Could you check a few things on this model? Use its own coordinates, in mm. A direction names the side the tool comes from. Give positions to 0.01 mm unless a question says otherwise; leave off trailing zeros. Loops run counter-clockwise (first coordinate to the right, second up) from the corner with the lowest first, then second, coordinate; pieces in that order, holes last. Notation, with made-up numbers: (-2.75, 61.5) - (12.25, 61.5) arc R19 ccw to (12.25, 98.5) - close; hole circle Ø6 at (50.25, -17.5). An arc over 180 degrees is marked (long way). Write each question's results on one line, items separated by ' | '. Start each with the question number.
(1) Suppose I cut it at B-B (z = 57.5). Please give me the cut outline in (x, y).
(2) Suppose I cut it at C-C (y = -56). Please give me the cut outline in (x, z).
(3) On a 3-axis mill with a long thin cutter (end or side, diameter ignored), from which of +Z, -Z, +X, -X, +Y, -Y can I reach the whole of each face in a straight line? I mean faces 4 (the face through (139.692, -45.148, 38.633)), 5 (the face through (-2, -88.9, 38)). Say none if no direction works.
(4) Suppose I cut it at A-A (x = -48.5). Please give me the cut outline in (y, z), and give its area (3 significant figures).
(5) For pin 1 (5 mm diameter, centred on y = -68.5, z = 16, fed in from -X); pin 2 (5 mm diameter, centred on y = -63.5, z = 19, fed in from +X); pin 3 (3 mm diameter, centred on y = -48, z = 56.5, fed in from -X), each with a flat end and sliding along its axis, tell me the tip position at first contact or that it passes through.
(6) I need wall thicknesses on line 1 (Y direction, x = -90, z = 25.5); line 2 (Y direction, x = -114.5, z = 46.5); line 3 (X direction, y = -73, z = 61.5). Which ranges of each line are inside material? Lowest first, please.
(7) If we mould it in two halves opening along X, with no side actions, what happens to faces 1 (the face through (-139.725, -75.533, 38.633)), 2 (the face through (-139.692, -43.752, 38.633)), 3 (the face through (2, 0, 39))? For each: released by +X, released by -X, zero draft, split by the parting line, or undercut.
from build123d import *

# Parameters (mm, degrees)
F1_DEPTH  = 76.2
F3_DEPTH  = 127
F4_DEPTH  = 127
F5_DEPTH  = 127
F6_DEPTH  = 127
F7_DEPTH  = 76.2
F8_DEPTH  = 76.2
F9_DEPTH  = 76.2
F10_DEPTH = 76.2


with BuildPart() as f1:
    # F0 (on Top) → F1 (new body)
    with BuildSketch(Plane.XY):
        Polygon((-152.4, -88.9), (0, -88.9), (152.4, -88.9), (152.4, 0), (0, 0), (-152.4, 0), align=None)
    extrude(amount=F1_DEPTH)

    # F2 (on face) → F3 (cut)
    with BuildSketch(Plane.XY.offset(76.2)):
        with BuildLine():
            Line((-152.4, -88.9), (-107.95, -88.9))
            ThreePointArc((-107.95, -88.9), (-139.380896, -75.880896), (-152.4, -44.45))
            Line((-152.4, -44.45), (-152.4, -88.9))
        make_face()
    extrude(amount=-F3_DEPTH, mode=Mode.SUBTRACT)

    # F2 (on face) → F4 (cut)
    with BuildSketch(Plane.XY.offset(76.2)):
        with BuildLine():
            ThreePointArc((-152.4, -44.45), (-139.380896, -75.880896), (-107.95, -88.9))
            Line((-107.95, -88.9), (-107.95, -76.2))
            ThreePointArc((-107.95, -76.2), (-139.7, -44.45), (-107.95, -12.7))
            Line((-107.95, -12.7), (-107.95, 0))
            Line((-107.95, 0), (-152.4, 0))
            Line((-152.4, 0), (-152.4, -44.45))
        make_face()
    extrude(amount=-F4_DEPTH, mode=Mode.SUBTRACT)

    # F2 (on face) → F5 (cut)
    with BuildSketch(Plane.XY.offset(76.2)):
        with BuildLine():
            ThreePointArc((107.95, 0), (139.380896, -13.019104), (152.4, -44.45))
            Line((152.4, -44.45), (152.4, 0))
            Line((152.4, 0), (107.95, 0))
        make_face()
    extrude(amount=-F5_DEPTH, mode=Mode.SUBTRACT)

    # F2 (on face) → F6 (cut)
    with BuildSketch(Plane.XY.offset(76.2)):
        with BuildLine():
            Line((107.95, -88.9), (152.4, -88.9))
            Line((152.4, -88.9), (152.4, -44.45))
            ThreePointArc((152.4, -44.45), (139.380896, -75.880896), (107.95, -88.9))
        make_face()
    extrude(amount=-F6_DEPTH, mode=Mode.SUBTRACT)

    # F2 (on face) → F7 (join)
    with BuildSketch(Plane.XY.offset(76.2)):
        with BuildLine():
            ThreePointArc((107.95, 0), (139.380896, -13.019104), (152.4, -44.45))
            Line((152.4, -44.45), (152.4, 0))
            Line((152.4, 0), (107.95, 0))
        make_face()
    extrude(amount=-F7_DEPTH)

    # F2 (on face) → F8 (join)
    with BuildSketch(Plane.XY.offset(76.2)):
        with BuildLine():
            ThreePointArc((-152.4, -44.45), (-139.380896, -75.880896), (-107.95, -88.9))
            Line((-107.95, -88.9), (-107.95, -76.2))
            ThreePointArc((-107.95, -76.2), (-139.7, -44.45), (-107.95, -12.7))
            Line((-107.95, -12.7), (-107.95, 0))
            Line((-107.95, 0), (-152.4, 0))
            Line((-152.4, 0), (-152.4, -44.45))
        make_face()
    extrude(amount=-F8_DEPTH)

    # F2 (on face) → F9 (cut)
    with BuildSketch(Plane.XY.offset(76.2)):
        with BuildLine():
            Line((0, -76.2), (107.95, -76.2))
            ThreePointArc((107.95, -76.2), (139.7, -44.45), (107.95, -12.7))
            Line((107.95, -12.7), (0, -12.7))
            Line((0, -12.7), (-107.95, -12.7))
            ThreePointArc((-107.95, -12.7), (-139.7, -44.45), (-107.95, -76.2))
            Line((-107.95, -76.2), (0, -76.2))
        make_face()
    extrude(amount=-F9_DEPTH, mode=Mode.SUBTRACT)

    # F2 (on face) → F10 (cut)
    with BuildSketch(Plane.XY.offset(76.2)):
        with BuildLine():
            Line((0, -76.2), (107.95, -76.2))
            ThreePointArc((107.95, -76.2), (139.7, -44.45), (107.95, -12.7))
            Line((107.95, -12.7), (0, -12.7))
            Line((0, -12.7), (-107.95, -12.7))
            ThreePointArc((-107.95, -12.7), (-139.7, -44.45), (-107.95, -76.2))
            Line((-107.95, -76.2), (0, -76.2))
        make_face()
    extrude(amount=-F10_DEPTH, mode=Mode.SUBTRACT)


solid = f1.part
Output values:
1) outline: (-152.4, -44.45) arc R44.45 ccw to (-107.95, -88.9) - (107.95, -88.9) arc R44.45 ccw to (152.4, -44.45) - (152.4, 0) - (-152.4, 0) - close; hole (-107.95, -76.2) - (107.95, -76.2) arc R31.75 ccw to (107.95, -12.7) - (-107.95, -12.7) arc R31.75 ccw to start
2) outline: (-150.87, 0) - (-137.52, 0) - (-137.52, 76.2) - (-150.87, 76.2) - close; (137.52, 0) - (150.87, 0) - (150.87, 76.2) - (137.52, 76.2) - close
3) face 4: +Z, -Z | face 5: +Z, -Z, +X, -X, -Y
4) outline: (-88.9, 0) - (-76.2, 0) - (-76.2, 76.2) - (-88.9, 76.2) - close; (-12.7, 0) - (0, 0) - (0, 76.2) - (-12.7, 76.2) - close | area: 1,940 mm2
5) pin 1: x = -146.83 | pin 2: x = 149.2 | pin 3: x = -152.35
6) line 1: -88.9 to -76.2, -12.7 to 0 | line 2: -88.41 to -75.52, -13.38 to 0 | line 3: -142.02 to -121.84, 121.84 to 142.02
7) face 1: released by -X | face 2: undercut | face 3: zero draft
